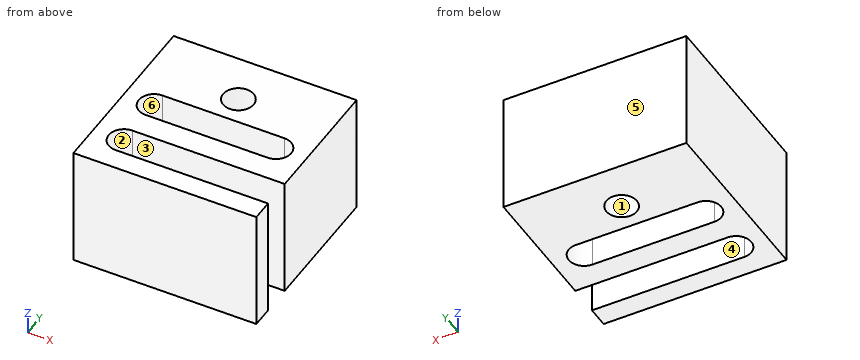
```python
from build123d import *

# Parameters (mm, degrees)
SKETCH1_W                   = 38.1
SKETCH1_H                   = 38.1
BOSS_EXTRUDE1_DEPTH         = 12.7
CUT_EXTRUDE1_DEPTH          = 25.4
F_1_4_0_25_DIAMETER_HOLE1_D = 6.35
CUT_EXTRUDE2_DEPTH          = 25.4


with BuildPart() as part:
    # Sketch1 → Boss-Extrude1 (new, symmetric)
    with BuildSketch(Plane.XY):
        Rectangle(SKETCH1_W, SKETCH1_H)
    extrude(amount=BOSS_EXTRUDE1_DEPTH, both=True)

    # Sketch2 → Cut-Extrude1 (cut)
    with BuildSketch(Plane.XY.offset(12.7)):
        with BuildLine():
            Line((-12.7, -8.255), (19.05, -8.255))
            ThreePointArc((19.05, -8.255), (22.225, -11.43), (19.05, -14.605))
            Line((19.05, -14.605), (-12.7, -14.605))
            ThreePointArc((-12.7, -14.605), (-15.875, -11.43), (-12.7, -8.255))
        make_face()
    extrude(amount=-CUT_EXTRUDE1_DEPTH, mode=Mode.SUBTRACT)

    # 1/4 (0.25) Diameter Hole1 (through all)
    with Locations(Plane.XY.offset(12.7)):
        with Locations((0, 8.89)):
            Hole(F_1_4_0_25_DIAMETER_HOLE1_D / 2)

    # Sketch7 → Cut-Extrude2 (cut)
    with BuildSketch(Plane.XY.offset(12.7)):
        with BuildLine():
            Line((-12.7, 3.175), (12.7, 3.175))
            ThreePointArc((12.7, 3.175), (15.875, 0), (12.7, -3.175))
            Line((12.7, -3.175), (-12.7, -3.175))
            ThreePointArc((-12.7, -3.175), (-15.875, 0), (-12.7, 3.175))
        make_face()
    extrude(amount=-CUT_EXTRUDE2_DEPTH, mode=Mode.SUBTRACT)


solid = part.part
```
Source: CAD feature listing. Evaluate the final solid. Frame: model axes, mm. Face numbers are marked on the shaded views. A direction names the side the tool comes from. Give positions to 0.01 mm unless a question says otherwise; leave off trailing zeros. Write each loop counter-clockwise with the first axis right and the second up, starting at its lowest first coordinate (ties: lowest second). Pieces come first, ordered by that corner, then holes.
1. Material intervals for line 1 along Y through (x, z) = (0, 7.25) (3 decimals); line 2 along Y through (x, z) = (10, -2) (3 decimals); line 3 along Y through (x, z) = (-15.5, 7.5), sorted ascending.
2. Access query for the marked faces 4, 5 and 6. Directions: +Z, -Z, +X, -X, +Y, -Y. A direction counts if a zero-diameter tool reaches every point of the face in a straight line with its end or side. Return the directions, or none.
3. Section query A-A (y = 8.89). Return the cut outline in (x, z) (3 decimals).
4. Pull-direction query (X, two-part tool) for the marked faces 1, 2 and 3; classes: +X half, -X half, draft (parallel to the pull), parting line (faces both ways), or undercut.
5. Section query D-D (x = 0). Return the cut outline in (y, z) (3 decimals).
6. Section query B-B (x = 4). Return the cut outline in (y, z) (3 decimals), then the cut area to 3 significant figures.
7. Section query C-C (z = 2.5). Return the cut outline in (x, y) (3 decimals).
Output values:
1. line 1: y = -19.05 to -14.605, -8.255 to -3.175, 3.175 to 5.715, 12.065 to 19.05
1. line 2: y = -19.05 to -14.605, -8.255 to -3.175, 3.175 to 19.05
1. line 3: y = -19.05 to -12.93, -9.93 to -1.5, 1.5 to 19.05
2. face 4: +Z, -Z, +X
2. face 5: +Z, -Z, +X, -X, +Y
2. face 6: +Z, -Z
3. outline: (-19.05, -12.7) - (-3.175, -12.7) - (-3.175, 12.7) - (-19.05, 12.7) - close; (3.175, -12.7) - (19.05, -12.7) - (19.05, 12.7) - (3.175, 12.7) - close
4. face 1: undercut
4. face 2: +X half
4. face 3: draft
5. outline: (-19.05, -12.7) - (-14.605, -12.7) - (-14.605, 12.7) - (-19.05, 12.7) - close; (-8.255, -12.7) - (-3.175, -12.7) - (-3.175, 12.7) - (-8.255, 12.7) - close; (3.175, -12.7) - (5.715, -12.7) - (5.715, 12.7) - (3.175, 12.7) - close; (12.065, -12.7) - (19.05, -12.7) - (19.05, 12.7) - (12.065, 12.7) - close
6. outline: (-19.05, -12.7) - (-14.605, -12.7) - (-14.605, 12.7) - (-19.05, 12.7) - close; (-8.255, -12.7) - (-3.175, -12.7) - (-3.175, 12.7) - (-8.255, 12.7) - close; (3.175, -12.7) - (19.05, -12.7) - (19.05, 12.7) - (3.175, 12.7) - close
6. area: 645 mm2
7. outline: (-19.05, -19.05) - (19.05, -19.05) - (19.05, -14.605) - (-12.7, -14.605) arc R3.175 cw to (-12.7, -8.255) - (19.05, -8.255) - (19.05, 19.05) - (-19.05, 19.05) - close; hole (-12.7, -3.175) - (12.7, -3.175) arc R3.175 ccw to (12.7, 3.175) - (-12.7, 3.175) arc R3.175 ccw to start; hole circle Ø6.35 at (0, 8.89)
